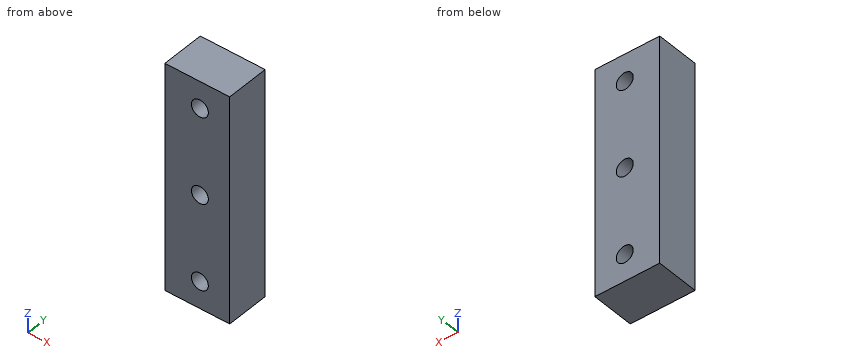
from build123d import *

# Parameters (mm, degrees)
BOSS_EXTRUDE1_DEPTH    = 12.7
F_10_CLEARANCE_HOLE1_D = 4.9784


with BuildPart() as part:
    # Sketch4 → Boss-Extrude1 (new body)
    with BuildSketch(Plane(origin=(0, 0, 0), x_dir=(1, 0, 0), z_dir=(0, 1, 0))):
        Polygon((-71.608792588, 6.232898137), (-71.608792588, 28.457898137), (-52.558792588, 28.457898137), (-52.558792588, -12.817101863), (-52.558792588, -38.217101863), (-71.608792588, -38.217101863), (-71.608792588, -12.817101863), align=None)
    extrude(amount=BOSS_EXTRUDE1_DEPTH)

    # #10 Clearance Hole1 (through all)
    with Locations(Plane(origin=(0, 12.7, 0), x_dir=(1, 0, 0), z_dir=(0, 1, 0))):
        with Locations((-61.333792588, 20.520398137), (-61.333792588, -4.879601863), (-61.333792588, -30.279601863)):
            Hole(F_10_CLEARANCE_HOLE1_D / 2)


solid = part.part
Geometry check sheet. Reference: the model listing, model coordinates, mm. Round coordinates to 2 decimals unless told otherwise and drop trailing zeros. Loops run counter-clockwise (first coordinate to the right, second up) from the corner with the lowest first, then second, coordinate; pieces in that order, holes last.
Item 1: Cross-section at B-B on y = 6. Record the boundary of the cut face in (x, z), then the cut area to 3 significant figures.
Item 2: Cross-section at A-A on z = 32. Record the boundary of the cut face in (x, y).
Item 3: Thickness scan on line 1 (Z direction, x = -60.25, y = 9); line 2 (X direction, y = 1.25, z = -18.5). Record the ranges inside material, lowest first.
Answer sheet:
1. outline: (-71.61, -28.46) - (-52.56, -28.46) - (-52.56, 38.22) - (-71.61, 38.22) - close; hole circle Ø4.98 at (-61.33, -20.52); hole circle Ø4.98 at (-61.33, 4.88); hole circle Ø4.98 at (-61.33, 30.28)
1. area: 1,210 mm2
2. outline: (-71.61, 0) - (-63.13, 0) - (-63.13, 12.7) - (-71.61, 12.7) - close; (-59.53, 0) - (-52.56, 0) - (-52.56, 12.7) - (-59.53, 12.7) - close
3. line 1: z = -28.46 to -22.76, -18.28 to 2.64, 7.12 to 28.04, 32.52 to 38.22
3. line 2: x = -71.61 to -62.79, -59.88 to -52.56
